Build history of the part. All positions in model axes, mm. A direction names the side the tool comes from. Round coordinates to 2 decimals unless told otherwise and drop trailing zeros. Write each loop counter-clockwise with the first axis right and the second up, starting at its lowest first coordinate (ties: lowest second). Pieces come first, ordered by that corner, then holes. Notation, with made-up numbers: M 87,-7 L 122,-7 A17 ccw 122,26 Z; hole C -8,-10 d6. An arc over 180 degrees is marked long. Use a Markdown table: item, result.
from build123d import *

# Parameters (mm, degrees)
BOSS_EXTRUDE2_DEPTH = 52.07
FILLET1_R           = 2.54
FILLET2_R           = 2.54
SKETCH2_R           = 2.487911977
CUT_EXTRUDE1_DEPTH  = 6.35
SKETCH3_R           = 2.511508717
CUT_EXTRUDE2_DEPTH  = 6.35
SKETCH4_R           = 2.535513074
SKETCH4_R_2         = 2.663596319
CUT_EXTRUDE3_DEPTH  = 6.35


with BuildPart() as part:
    # Sketch1 → Boss-Extrude2 (new body)
    with BuildSketch(Plane.XY):
        Polygon((-26.962285336, 42.108267604), (-26.962285336, -25.93406259), (49.683796158, -25.93406259), (31.840285665, -11.333620206), (30.474759276, -12.836120693), (-15.063657258, 28.550827293), (-13.698130869, 30.053327779), align=None)
        Polygon((-23.192135268, -21.36418372), (-23.192135268, 31.68438668), (35.177665187, -21.36418372), align=None, mode=Mode.SUBTRACT)
    extrude(amount=BOSS_EXTRUDE2_DEPTH)

    # Fillet1
    fillet1_edges = [part.edges().sort_by_distance(p)[0] for p in [
        (49.683796158, -25.93406259, 26.035),
        (-26.962285336, 42.108267604, 26.035),
    ]]
    fillet(fillet1_edges, radius=FILLET1_R)

    # Fillet2
    fillet2_edges = [part.edges().sort_by_distance(p)[0] for p in [
        (-26.962285336, -25.93406259, 26.035),
    ]]
    fillet(fillet2_edges, radius=FILLET2_R)

    # Sketch2 → Cut-Extrude1 (cut)
    with BuildSketch(Plane(origin=(8.761925392, 9.640822229, 0), x_dir=(0.7400339952176945, -0.6725694654993916, 0), z_dir=(0.6725694654993916, 0.7400339952176945, 0))):
        with Locations(Location((-36.410725244, -45.039764093, 0), (0, 0, 180))):
            Circle(SKETCH2_R)
        with Locations(Location((-36.342932428, -37.794805414, 0), (0, 0, 180))):
            Circle(SKETCH2_R)
        with Locations(Location((-36.113890977, -14.695763967, 0), (0, 0, 180))):
            Circle(SKETCH2_R)
        with Locations(Location((-36.113890977, -7.677508428, 0), (0, 0, 180))):
            Circle(SKETCH2_R)
        with Locations(Location((38.19748483, -45.003751016, 0), (0, 0, 180))):
            Circle(SKETCH2_R)
        with Locations(Location((38.265277646, -37.758792337, 0), (0, 0, 180))):
            Circle(SKETCH2_R)
        with Locations(Location((38.494319097, -14.659750891, 0), (0, 0, 180))):
            Circle(SKETCH2_R)
        with Locations(Location((38.494319097, -7.641495351, 0), (0, 0, 180))):
            Circle(SKETCH2_R)
    extrude(amount=-CUT_EXTRUDE1_DEPTH, mode=Mode.SUBTRACT)

    # Sketch3 → Cut-Extrude2 (cut)
    with BuildSketch(Plane(origin=(7.214216448, 8.816647023, 0), x_dir=(0.773931651192209, -0.6332691365311442, 0), z_dir=(0.6332691365311442, 0.773931651192209, 0))):
        with Locations(Location((37.297632804, -37.151246131, 0), (0, 0, 180))):
            Circle(SKETCH3_R)
        with Locations(Location((37.407323838, -44.063868687, 0), (0, 0, 180))):
            Circle(SKETCH3_R)
    extrude(amount=-CUT_EXTRUDE2_DEPTH, mode=Mode.SUBTRACT)

    # Sketch4 → Cut-Extrude3 (cut)
    with BuildSketch(Plane(origin=(7.214216448, 8.816647023, 0), x_dir=(0.773931651192209, -0.6332691365311442, 0), z_dir=(0.6332691365311442, 0.773931651192209, 0))):
        with Locations(Location((37.100504768, -5.630572581, 0), (0, 0, 180))):
            Circle(SKETCH4_R)
        with Locations(Location((37.232498306, -12.582232269, 0), (0, 0, 180))):
            Circle(SKETCH4_R_2)
    extrude(amount=-CUT_EXTRUDE3_DEPTH, mode=Mode.SUBTRACT)


solid = part.part
Q1. Two-plate mould, pull along Z, no slides. Class faces 1 (the flat face through (9, 4, 0)), 2 (the cylindrical face through (-21.351, 33.731, 15.443)), 3 (the flat face through (38.095, -16.452, 25.671)): +Z half, -Z half, draft (parallel to the pull), parting line (faces both ways), or undercut.
Response values:
| item | result |
|---|---|
| face 1 | -Z half |
| face 2 | undercut |
| face 3 | draft |
Q2. Drop flat-ended pins along their axis: P1, Ø8, axis at x = -13.5, z = 37, coming from the +Y side; P2, Ø5, axis at y = 27, z = 28.5, coming from the +X side; P3, Ø1.5, axis at y = 25, z = 40.5, coming from the +X side. Give the stop position or say it passes through.
Response values:
| item | result |
|---|---|
| P1 | stops at y = 33.28 |
| P2 | stops at x = -10.61 |
| P3 | stops at x = -10.33 |
Q3. Which spindle directions (+Z, -Z, +X, -X, +Y, -Y) get a long thin tool onto all of the face, cutting with end or side? Do faces 4 (the flat face through (37.765, -16.718, 38.347)), 5 (the cylindrical face through (44.946, -24.289, 26.399)). Say none if no direction does.
Response values:
| item | result |
|---|---|
| face 4 | none |
| face 5 | +Z, -Z, +X |
Q4. Cut at B-B on y = -5.5. Give the cut face in (x, z).
Response values:
| item | result |
|---|---|
| outline | M -26.96,0 L -23.19,0 L -23.19,52.07 L -26.96,52.07 Z; M 17.72,0 L 22.4,0 L 22.4,52.07 L 17.72,52.07 Z |
Q5. Drill centre lines: L1, parallel to X at y = -17.5, z = 6; L2, parallel to X at y = 9, z = 46; L3, parallel to Y at x = -18.5, z = 29. Where is each one in solid material? Low to high.
Response values:
| item | result |
|---|---|
| L1 | x = -26.96 to -23.19, 38.63 to 39.38 |
| L2 | x = -26.96 to -23.19, 1.77 to 6.45 |
| L3 | y = -25.93 to -21.36, 27.42 to 34.42 |
Q6. Cut at A-A on z = 19. Give the cut face in (x, y), and give its area (3 significant figures).
Response values:
| item | result |
|---|---|
| outline | M -26.96,-23.39 A2.54 ccw -24.42,-25.93 L 42.57,-25.93 A2.54 ccw 44.18,-21.43 L 31.84,-11.33 L 30.47,-12.84 L -15.06,28.55 L -13.7,30.05 L -22.71,38.25 A2.54 ccw -26.96,36.37 Z; hole M -23.19,-21.36 L 35.18,-21.36 L -23.19,31.68 Z |
| area | 868 mm2 |
Q7. Cut at C-C on x = -10.5. Give the cut face in (y, z).
Response values:
| item | result |
|---|---|
| outline | M -25.93,0 L -21.36,0 L -21.36,52.07 L -25.93,52.07 Z; M 20.15,0 L 24.4,0 L 24.4,52.07 L 20.15,52.07 Z |
